Could you check a few things on this model? Use its own coordinates, in mm. Face numbers are marked on the shaded views. A direction names the side the tool comes from. Coordinates: 2 decimals unless noted, no trailing zeros. Loops run counter-clockwise (first coordinate to the right, second up) from the corner with the lowest first, then second, coordinate; pieces in that order, holes last. Notation, with made-up numbers: (-26.75, -35.5) - (7.25, -35.5) arc R16 ccw to (7.25, -10.5) - close; hole circle Ø10 at (60.5, -24). An arc over 180 degrees is marked (long way). Use CSV: the item, a comma, the result in double quotes.
from build123d import *

# Parameters (mm, degrees)
SKETCH_1_R      = 24.5
EXTRUDE_1_DEPTH = 4
SKETCH_Q_R      = 60
EXTRUDE_2_DEPTH = 5
SKETCH_3_R      = 17.5
EXTRUDE_3_DEPTH = 150
SKETCH_4_R      = 100
EXTRUDE_4_DEPTH = 10
CHAMFER_1_SIZE  = 45
CHAMFER_2_SIZE  = 30
CHAMFER_2_SIZE2 = 51.961524227


with BuildPart() as part:
    # 草图1 → 凸台-拉伸1 (new body)
    with BuildSketch(Plane(origin=(0, 0, 0), x_dir=(1, 0, 0), z_dir=(0, 1, 0))):
        with Locations(Location((0, 0, 0), (0, 0, 270))):
            Circle(SKETCH_1_R)
    extrude(amount=EXTRUDE_1_DEPTH)

    # q → 凸台-拉伸2 (add)
    with BuildSketch(Plane(origin=(0, 4, 0), x_dir=(1, 0, 0), z_dir=(0, 1, 0))):
        with Locations(Location((0, 0, 0), (0, 0, 270))):
            Circle(SKETCH_Q_R)
    extrude(amount=EXTRUDE_2_DEPTH)

    # 草图3 → 凸台-拉伸3 (add)
    with BuildSketch(Plane(origin=(0, 9, 0), x_dir=(1, 0, 0), z_dir=(0, 1, 0))):
        with Locations(Location((0, 0, 0), (0, 0, 270))):
            Circle(SKETCH_3_R)
    extrude(amount=EXTRUDE_3_DEPTH)

    # 草图4 → 凸台-拉伸4 (add)
    with BuildSketch(Plane(origin=(0, 159, 0), x_dir=(1, 0, 0), z_dir=(0, 1, 0))):
        with Locations(Location((0, 0, 0), (0, 0, 270))):
            Circle(SKETCH_4_R)
    extrude(amount=EXTRUDE_4_DEPTH)

    # 倒角1
    # the kernel refuses this chamfer: 45 mm, written as the material it adds along each edge
    with BuildSketch(Plane(origin=(0, 9, 0), x_dir=(0, 0, 1), z_dir=(-1, 0, 0))) as chamfer_1_piece_1_section:
        Polygon((17.5, CHAMFER_1_SIZE), (17.5 + CHAMFER_1_SIZE, 0), (17.5, 0), align=None)
    chamfer_1_piece_1 = revolve(axis=Axis((0, 9, 0), (0, 1, 0)), mode=Mode.PRIVATE)
    chamfer_1_piece_1 = chamfer_1_piece_1 & Plane(origin=(0, 32.95787502, 0), x_dir=(0, 0, 1), z_dir=(0, -1, 0)) * Cylinder(60, 250, mode=Mode.PRIVATE)
    add(chamfer_1_piece_1)

    # 倒角2
    chamfer_2_edges = [part.edges().sort_by_distance(p)[0] for p in [
        (0, 159, -17.5),
    ]]
    chamfer_2_side = [part.faces().sort_by_distance(p)[0] for p in [
        (0, 106.5, -17.5),
    ]]
    chamfer(chamfer_2_edges, length=CHAMFER_2_SIZE, length2=CHAMFER_2_SIZE2, reference=chamfer_2_side[0])


solid = part.part
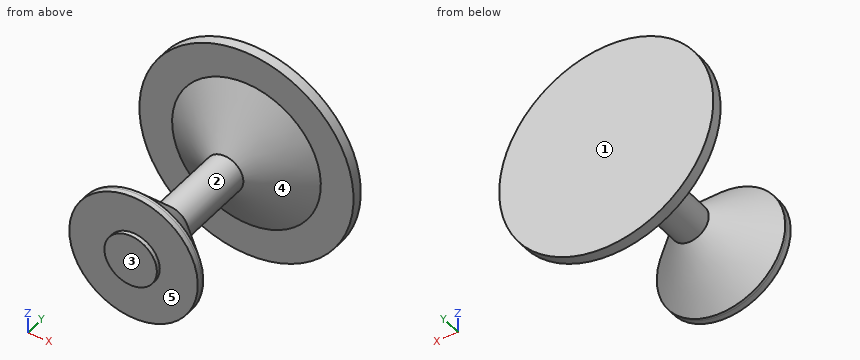
(1) Will these pins go through, and if not, where does the flat tip stop? pin 1 (1.5 mm diameter, centred on x = -42, z = -34, fed in from -Y); pin 2 (12 mm diameter, centred on y = 136.5, z = 4, fed in from -X); pin 3 (12 mm diameter, centred on x = -17.5, y = 122.5, fed in from +Z).
Computed:
pin 1,"stops at y = 4"
pin 2,"stops at x = -40.7"
pin 3,"stops at z = 13.19"
(2) Suppose I cut it at B-B (x = 0). Write out the boundary of the cut face in (y, z), plus the area to 3 significant figures.
Computed:
outline,"(0, -24.5) - (4, -24.5) - (4, -60) - (11.5, -60) - (54, -17.5) - (129, -17.5) - (159, -69.46) - (159, -100) - (169, -100) - (169, 100) - (159, 100) - (159, 69.46) - (129, 17.5) - (54, 17.5) - (11.5, 60) - (4, 60) - (4, 24.5) - (0, 24.5) - close"
area,"11,600 mm²"
(3) Suppose I cut it at A-A (z = 0). Write out the boundary of the cut face in (x, y), plus the area to 3 significant figures.
Computed:
outline,"(-100, 159) - (-69.46, 159) - (-17.5, 129) - (-17.5, 54) - (-60, 11.5) - (-60, 4) - (-24.5, 4) - (-24.5, 0) - (24.5, 0) - (24.5, 4) - (60, 4) - (60, 11.5) - (17.5, 54) - (17.5, 129) - (69.46, 159) - (100, 159) - (100, 169) - (-100, 169) - close"
area,"11,600 mm²"
(4) Which directions (+Z, -Z, +X, -X, +Y, -Y) give clear straight access to the entire face, cutting with the end or side of a thin tool? Please do the marked faces 4 and 5.
Computed:
face 4,"none"
face 5,"-Y"
(5) Thinking about a two-plate mould opening in Y: for the marked faces 1, 2 and 3, which applies, +Y half, -Y half, draft (parallel to the pull), parting line (faces both ways), or undercut?
Computed:
face 1,"+Y half"
face 2,"undercut"
face 3,"-Y half"
(6) Suppose I cut it at D-D (z = -82). Write out the boundary of the cut face in (x, y).
Computed:
outline,"(-57.24, 159) - (57.24, 159) - (57.24, 169) - (-57.24, 169) - close"
(7) Please list where these lines run through material, in increasing order: line 1 (Y direction, x = -41, z = 83); line 2 (Y direction, x = -16, z = 44); line 3 (Y direction, x = -13, z = 23).
Computed:
line 1,"y = 159 to 169"
line 2,"y = 4 to 24.68, 145.93 to 169"
line 3,"y = 4 to 45.08, 134.15 to 169"
(8) Suppose I cut it at C-C (y = 91). Write out the boundary of the cut face in (x, z), plus the area to 3 significant figures.
Computed:
outline,"circle Ø35 at (0, 0)"
area,"962 mm²"
